Autodesk Inventor part; units mm, degrees
ref_plane "Work Plane1" through (0, 19.05, 0) normal (0, 1, 0) x (-1, 0, 0)
ref_plane "YZ Plane" through (0, 0, 0) normal (1, 0, 0) x (0, 1, 0)
ref_plane "XY Plane" through (0, 0, 0) normal (0, 0, 1) x (1, 0, 0)
sketch "Sketch1" plane through (0, 0, 0) normal (0, 1, 0) x (-1, 0, 0)
  line L0 (-12.7, 12.7) -> (-12.7, -12.7)
  line L1 (-12.7, -12.7) -> (12.7, -12.7)
  line L2 (12.7, -12.7) -> (12.7, 12.7)
  line L3 (12.7, 12.7) -> (-12.7, 12.7)
  line L4 (-12.7, 12.7) -> (12.7, -12.7) construction
  line L5 (-12.7, -12.7) -> (12.7, 12.7) construction
  point P0 (0, 0)
  dimension "base" = 25.4
ref_plane "Work Plane1" through (0, 19.05, 0) normal (0, 1, 0) x (-1, 0, 0)
sketch "Sketch2" plane through (0, 19.05, 0) normal (0, 1, 0) x (-1, 0, 0)
  line L0 (-5.08, 5.08) -> (-5.08, -5.08)
  line L1 (-5.08, -5.08) -> (5.08, -5.08)
  line L2 (5.08, -5.08) -> (5.08, 5.08)
  line L3 (5.08, 5.08) -> (-5.08, 5.08)
  line L4 (-5.08, 5.08) -> (5.08, -5.08) construction
  line L5 (-5.08, -5.08) -> (5.08, 5.08) construction
  point P0 (0, 0)
  dimension "topOfPyramid" = 10.16
loft "Loft1" add profiles "Sketch1", "Sketch2"
sketch "Sketch3" plane through (0, 0, 0) normal (0, 0, 1) x (1, 0, 0)
  arc A0 (-3.81, 24.13) -> (3.81, 24.13) centre (0, 24.13) ccw
  arc A1 (-5.08, 24.13) -> (5.08, 24.13) centre (0, 24.13) ccw
  line L0 (5.08, 19.05) -> (-5.08, 19.05)
  line L1 (3.81, 24.13) -> (5.08, 24.13)
  line L2 (-3.81, 24.13) -> (-5.08, 24.13)
  line L3 (-5.08, 24.13) -> (-5.08, 19.05)
  line L4 (5.08, 24.13) -> (5.08, 19.05)
  line L5 (12.7, 0) -> (5.08, 19.05)
  line L6 (5.08, 19.05) -> (0, 19.05)
  line L7 (-5.08, 19.05) -> (5.08, 19.05)
  line L8 (-5.08, 19.05) -> (0, 19.05)
  point P0 (0, 0)
  dimension "innerDiamForRope" = 7.62
  dimension "centerForRope" = 5.08
  dimension "outsideDiam" = 10.16
extrude "Extrusion1" add sketch "Sketch3" along normal mid plane 10.16
fillet "Fillet3" radius 1.5875 4 edges at (8.89, 9.525, 8.89) (8.89, 9.525, -8.89) (-8.89, 9.525, 8.89) (-8.89, 9.525, -8.89)
fillet "Fillet5" radius 0.7937 2 edges at (0, 20.32, 5.08) (0, 20.32, -5.08)
equation "\"centerForRope\" = 0.5 * outsideDiam"
equation "\"widthOfTop\" = topOfPyramid"
properties part number "SupportForMouseWire"
Here's how the part is built. I have some questions about the finished solid (model axes, mm). Give positions to 0.01 mm unless a question says otherwise; leave off trailing zeros.
(1) Thinking about a two-plate mould opening in X: for faces 1 (the face through (0.08, 20.32, -0.06)), 2 (the face through (0.4, 19.3, 5.08)), 3 (the face through (5.08, 22, 0)), 4 (the face through (-5.08, 22, 0)), which applies, pulls with the +X half, pulls with the -X half, needs draft (parallel to the pull), parting line crosses it, or undercut?
Output values:
face 1: undercut
face 2: needs draft
face 3: pulls with the +X half
face 4: pulls with the -X half
(2) Will these pins go through, and if not, where does the flat tip stop? pin 1 (1 mm diameter, centred on y = 9, z = -9, fed in from -X); pin 2 (6.5 mm diameter, centred on x = 2.5, y = 22, fed in from -Z); pin 3 (6 mm diameter, centred on x = 7, y = 21, fed in from -Z).
Output values:
pin 1: stops at x = -8.97
pin 2: stops at z = -5.2
pin 3: stops at z = -5.08
(3) If I drill on L1, parallel to X at y = 8.75, z = -2.75; L2, parallel to Y at x = 7, z = -11; L3, parallel to Y at x = 7.25, z = 7.25, over which ranges is the centre line in solid material (lowest first)?
Output values:
L1: x = -9.2 to 9.2
L2: y = 0 to 4.25
L3: y = 0 to 12.57
